from build123d import *

# Parameters (mm, degrees)
BOSS_EXTRUDE1_DEPTH     = 12.7
SKETCH4_R               = 2.5273
CUT_EXTRUDE1_DEPTH      = 13.5636
SKETCH5_R               = 3.81
CUT_EXTRUDE2_DEPTH      = 1
CUT_EXTRUDE2_DEPTH_BACK = 26.4
SKETCH6_R               = 8.128
SKETCH6_R_2             = 5.588
SKETCH6_R_3             = 6.604
SKETCH6_R_4             = 6.5532
CUT_EXTRUDE3_DEPTH      = 12.7
SKETCH7_W               = 4.7752
SKETCH7_H               = 38.5064
SKETCH7_W_2             = 7.874
SKETCH7_H_2             = 18.415
SKETCH7_W_3             = 4.826
SKETCH7_H_3             = 38.608
CUT_EXTRUDE4_DEPTH      = 12.7
SKETCH8_R               = 5.588
CUT_EXTRUDE5_DEPTH      = 6.35


with BuildPart() as part:
    # Sketch1 → Boss-Extrude1 (new body, symmetric)
    with BuildSketch(Plane(origin=(0, 0, 0), x_dir=(1, 0, 0), z_dir=(0, 1, 0))):
        with BuildLine():
            Line((-116.078, -5.08), (-116.078, -11.3538))
            ThreePointArc((-116.078, -11.3538), (-114.590102448, -14.945902448), (-110.998, -16.4338))
            Line((-110.998, -16.4338), (-95.758, -16.4338))
            ThreePointArc((-95.758, -16.4338), (-92.165897552, -14.945902448), (-90.678, -11.3538))
            Line((-90.678, -11.3538), (-90.678, -5.08))
            ThreePointArc((-90.678, -5.08), (-89.190102448, -1.487897552), (-85.598, 0))
            Line((-85.598, 0), (-10, 0))
            Line((-10, 0), (0, -10))
            Line((0, -10), (0, -183.7766))
            Line((0, -183.7766), (-10, -193.7766))
            Line((-10, -193.7766), (-196.756, -193.7766))
            Line((-196.756, -193.7766), (-206.756, -183.7766))
            Line((-206.756, -183.7766), (-206.756, -10))
            Line((-206.756, -10), (-196.756, 0))
            Line((-196.756, 0), (-121.158, 0))
            ThreePointArc((-121.158, 0), (-117.565897552, -1.487897552), (-116.078, -5.08))
        make_face()
    extrude(amount=BOSS_EXTRUDE1_DEPTH, both=True)

    # Sketch4 → Cut-Extrude1 (cut)
    with BuildSketch(Plane(origin=(0, 0, 0), x_dir=(0, 0, -1), z_dir=(1, 0, 0))):
        with Locations((-39.3573, -0.2032)):
            Circle(SKETCH4_R)
        with Locations((-154.4193, -0.2032)):
            Circle(SKETCH4_R)
    cut_extrude1 = extrude(amount=-CUT_EXTRUDE1_DEPTH, mode=Mode.SUBTRACT)

    # Mirror1: Cut-Extrude1 across plane
    add(cut_extrude1.mirror(Plane(origin=(-103.378, 0, 0), x_dir=(0, 0, 1), z_dir=(1, 0, 0))), mode=Mode.SUBTRACT)

    # Sketch5 → Cut-Extrude2 (cut, two sides)
    with BuildSketch(Plane(origin=(0, 12.7, 0), x_dir=(1, 0, 0), z_dir=(0, 1, 0))) as cut_extrude2_sk:
        with Locations((-196.7484, -10.0076)):
            Circle(SKETCH5_R)
        with Locations((-161.5948, -10.0076)):
            Circle(SKETCH5_R)
        with Locations((-125.5014, -10.0076)):
            Circle(SKETCH5_R)
        with Locations((-81.2546, -10.0076)):
            Circle(SKETCH5_R)
        with Locations((-9.906, -183.769)):
            Circle(SKETCH5_R)
        with Locations((-46.101, -183.769)):
            Circle(SKETCH5_R)
        with Locations((-81.2546, -183.769)):
            Circle(SKETCH5_R)
        with Locations((-125.5014, -183.769)):
            Circle(SKETCH5_R)
        with Locations((-161.5948, -183.769)):
            Circle(SKETCH5_R)
        with Locations((-196.7484, -183.769)):
            Circle(SKETCH5_R)
        with Locations((-9.906, -53.467)):
            Circle(SKETCH5_R)
        with Locations((-9.906, -97.8154)):
            Circle(SKETCH5_R)
        with Locations((-9.906, -140.3096)):
            Circle(SKETCH5_R)
        with Locations((-196.85, -53.467)):
            Circle(SKETCH5_R)
        with Locations((-196.85, -97.8154)):
            Circle(SKETCH5_R)
        with Locations((-196.85, -140.3096)):
            Circle(SKETCH5_R)
        with Locations((-46.101, -10.0076)):
            Circle(SKETCH5_R)
        with Locations((-9.906, -10.0076)):
            Circle(SKETCH5_R)
    extrude(amount=CUT_EXTRUDE2_DEPTH, mode=Mode.SUBTRACT)
    extrude(cut_extrude2_sk.sketch, amount=-CUT_EXTRUDE2_DEPTH_BACK, mode=Mode.SUBTRACT)

    # Sketch6 → Cut-Extrude3 (cut)
    with BuildSketch(Plane(origin=(0, 12.7, 0), x_dir=(1, 0, 0), z_dir=(0, 1, 0))):
        with Locations((-177.038, -45.5676)):
            Circle(SKETCH6_R)
        with Locations((-173.482, -96.7232)):
            Circle(SKETCH6_R_2)
        with Locations((-178.562, -148.8186)):
            Circle(SKETCH6_R_3)
        with Locations((-28.2321, -45.5676)):
            Circle(SKETCH6_R_4)
        with Locations((-33.2994, -96.7232)):
            Circle(SKETCH6_R_2)
        with Locations((-29.4386, -148.8186)):
            Circle(SKETCH6_R)
    extrude(amount=-CUT_EXTRUDE3_DEPTH, mode=Mode.SUBTRACT)

    # Sketch7 → Cut-Extrude4 (cut)
    with BuildSketch(Plane.XZ.offset(12.7)):
        with Locations((-175.6664, 53.467)):
            Rectangle(SKETCH7_W, SKETCH7_H)
        with Locations((-174.78756, 97.8154)):
            Rectangle(SKETCH7_W_2, SKETCH7_H_2)
        with Locations((-175.641, 140.3096)):
            Rectangle(SKETCH7_W_3, SKETCH7_H_3)
        with Locations((-31.115, 140.3096)):
            Rectangle(SKETCH7_W_3, SKETCH7_H_3)
        with Locations((-31.0896, 53.467)):
            Rectangle(SKETCH7_W, SKETCH7_H)
        with Locations((-31.96844, 97.8154)):
            Rectangle(SKETCH7_W_2, SKETCH7_H_2)
    extrude(amount=-CUT_EXTRUDE4_DEPTH, mode=Mode.SUBTRACT)

    # Sketch8 → Cut-Extrude5 (cut)
    with BuildSketch(Plane.XZ.offset(12.7)):
        with Locations((-191.5414, 119.0244)):
            Circle(SKETCH8_R)
        with Locations((-191.5414, 74.7522)):
            Circle(SKETCH8_R)
        with Locations((-15.2146, 74.7522)):
            Circle(SKETCH8_R)
        with Locations((-15.2146, 119.0244)):
            Circle(SKETCH8_R)
    extrude(amount=-CUT_EXTRUDE5_DEPTH, mode=Mode.SUBTRACT)


solid = part.part
The model under review builds one solid part; all positions refer to its coordinate system, in mm. A direction names the side the tool comes from. Give positions to 0.01 mm unless a question says otherwise; leave off trailing zeros. Order: outer loops, then holes, each group sorted by start corner. A loop starts at its lowest first (then second) coordinate and runs counter-clockwise, first axis right, second up. Notation, with made-up numbers: M 36.5,81 L 48.5,81 A21 cw 48.5,111 Z; hole C 83.25,83 d8. An arc over 180 degrees is marked long. Answer in a Markdown table with one row per item. Add a question column.
1. For pin 1 Ø10 at (x, z) = (-191.54, 119.02) entering from -Y; pin 2 Ø2.5 at (x, z) = (-174, 104.5) entering from -Y, all flat-tipped, find the tip position at first contact; note any pin that passes through.
2. Mouldability with a two-part tool opening along Y and no side actions: class faces 6 (the cylindrical face through (-197.68, 0.18, 144.03)), 7 (the flat face through (-13.564, 0, 154)), 8 (the flat face through (-176, 0, 90)) as released by +Y, released by -Y, zero draft, split by the parting line, or undercut.
3. Add section B-B on y = -9.5. Count the separate pieces of the cut face and the enclosed holes in it, plus the area to 3 significant figures.
4. Add section A-A on x = -190. State the section outline as (y, z) points.
5. Machinability: for faces 1 (the flat face through (-90.678, 0, 8)), 2 (the flat face through (-193.192, 0, 39)), 3 (the flat face through (-159, 0, 0)), 4 (the flat face through (-33.528, -6, 140)), 5 (the cylindrical face through (-197.57, 0.18, 187.49)), which of the approach directions +Z, -Z, +X, -X, +Y, -Y give a long, thin tool a straight path to every point of the face, cutting with its end or side? Answer none if there is none.
6. To check wall thickness, follow line 1 along X through (y, z) = (10.5, 45.5); line 2 along X through (y, z) = (6.5, 140); line 3 along Z through (x, y) = (-126, -5). State the ranges of each line that lie inside material, in increasing order.
The answers:
| question | item | result |
|---|---|---|
| 1 | pin 1 | y = -6.35 |
| 1 | pin 2 | y = 0 |
| 2 | face 6 | zero draft |
| 2 | face 7 | undercut |
| 2 | face 8 | released by -Y |
| 3 | separate pieces | 1 |
| 3 | enclosed holes | 28 |
| 3 | area | 37,200 mm2 |
| 4 | outline | M -12.7,0 L 12.7,0 L 12.7,193.78 L -12.7,193.78 L -12.7,124.4 L -6.35,124.4 L -6.35,113.65 L -12.7,113.65 L -12.7,80.12 L -6.35,80.12 L -6.35,69.38 L -12.7,69.38 Z |
| 5 | face 1 | -Z, +Y, -Y |
| 5 | face 2 | -X |
| 5 | face 3 | -Z, +X, -X, +Y, -Y |
| 5 | face 4 | -Y |
| 5 | face 5 | +Y, -Y |
| 6 | line 1 | -206.76 to -185.17, -168.91 to -34.78, -21.68 to 0 |
| 6 | line 2 | -206.76 to -200.65, -193.05 to -13.7, -6.11 to 0 |
| 6 | line 3 | 0 to 6.23, 13.78 to 179.99, 187.55 to 193.78 |
